The model under review builds one solid part; all positions refer to its coordinate system, in mm. A direction names the side the tool comes from. Coordinates: 2 decimals unless noted, no trailing zeros. Write each loop counter-clockwise with the first axis right and the second up, starting at its lowest first coordinate (ties: lowest second). Pieces come first, ordered by that corner, then holes. Notation, with made-up numbers: (84, 82.5) - (100, 82.5) arc R23 ccw to (100, 117.5) - close; hole circle Ø4 at (75, 23.25). An arc over 180 degrees is marked (long way). Put each result on its own line as item: value.
from build123d import *

# Parameters (mm, degrees)
SKETCH2_R           = 2.95
SKETCH2_R_2         = 8.099999999
BOSS_EXTRUDE1_DEPTH = 1


with BuildPart() as part:
    # Sketch1 → Revolve1 (revolve)
    with BuildSketch(Plane(origin=(0, 0, 0), x_dir=(0, 0, -1), z_dir=(1, 0, 0))):
        Polygon((18, 2.05), (18, 2.4), (17.5, 2.9), (8, 2.9), (8, 4), (0, 4), (0, 2.05), align=None)
    revolve(axis=Axis((0, 0, 0), (0, 0, -1)))

    # Sketch2 → Boss-Extrude1 (add)
    with BuildSketch(Plane(origin=(0, 0, -8), x_dir=(-1, 0, 0), z_dir=(0, 0, -1))):
        with BuildLine():
            Line((9.857790067, 21.711729889), (12.493283293, 10.967026744))
            Line((12.493283293, 10.967026744), (4.275989158, -2.59150858))
            ThreePointArc((4.275989158, -2.59150858), (-2.59150858, -4.275989158), (-4.275989158, 2.59150858))
            Line((-4.275989158, 2.59150858), (-0.302187827, 9.148280777))
            ThreePointArc((-0.302187827, 9.148280777), (-7.892239666, 25.676183207), (9.857790067, 21.711729889))
        make_face()
        Circle(SKETCH2_R, mode=Mode.SUBTRACT)
        with Locations((0, 19.293781382)):
            Circle(SKETCH2_R_2, mode=Mode.SUBTRACT)
    extrude(amount=BOSS_EXTRUDE1_DEPTH)


solid = part.part
1. Consider section B-B on y = 0. State the section outline as (x, z) points.
Determined:
outline: (-5.85, -9) - (-2.95, -9) - (-2.95, -8) - (-2.9, -8) - (-2.9, -17.5) - (-2.4, -18) - (-2.05, -18) - (-2.05, 0) - (-4, 0) - (-4, -8) - (-5.85, -8) - close; (2.05, -18) - (2.4, -18) - (2.9, -17.5) - (2.9, -8) - (2.95, -8) - (2.95, -9) - (5, -9) - (5, -8) - (4, -8) - (4, 0) - (2.05, 0) - close
2. Consider section A-A on x = 7.5. State the section outline as (y, z) points.
Determined:
outline: (12.45, -9) - (16.23, -9) - (16.23, -8) - (12.45, -8) - close; (22.35, -9) - (26.13, -9) - (26.13, -8) - (22.35, -8) - close
3. Machinability: for faces 1 (the cylindrical face through (0.1, -2.9, -12.7)), 2 (the flat face through (-11.16, 16.41, -8.49)), 3 (the cylindrical face through (-3.905, -0.867, -3.944)), which of the approach directions +Z, -Z, +X, -X, +Y, -Y give a long, thin tool a straight path to every point of the face, cutting with its end or side? Answer none if there is none.
Determined:
face 1: -Z
face 2: +Z, -Z, -X, +Y
face 3: +Z
4. To check wall thickness, follow probe 1 along X at (y, z) = (0, -3.75); probe 2 along X at (y, z) = (0, -14); probe 3 along Z at (x, y) = (-4.5, 4.5). State the ranges of each line that lie inside material, in increasing order.
Determined:
probe 1: x = -4 to -2.05, 2.05 to 4
probe 2: x = -2.9 to -2.05, 2.05 to 2.9
probe 3: z = -9 to -8
5. For pin 1 Ø1.5 at (x, y) = (5.5, 25) entering from +Z; pin 2 Ø2 at (x, z) = (4, -6) entering from +Y; pin 3 Ø6 at (x, z) = (1.5, -14.5) entering from -Y; pin 4 Ø2.5 at (x, y) = (0, 0) entering from -Z, all flat-tipped, find the tip position at first contact; note any pin that passes through.
Determined:
pin 1: stops at z = -8
pin 2: stops at y = 2.65
pin 3: stops at y = -2.9
pin 4: passes through
6. Consider section D-D on y = 20.5. State the section outline as (x, z) points (3 decimals), plus the area to 3 significant figures.
Determined:
outline: (-10.155, -9) - (-8.01, -9) - (-8.01, -8) - (-10.155, -8) - close; (8.01, -9) - (10.078, -9) - (10.078, -8) - (8.01, -8) - close
area: 4.21 mm^2
7. The part is to be moulded in two halves that separate along X. For faces 4 (the flat face through (1, -2, -18)), 5 (the cylindrical face through (1.054, 27.325, -8.493)), 6 (the cylindrical face through (2.033, -0.267, -9.126)), 7 (the flat face through (2.32, 5.82, -8.49)), say which applies: +X half, -X half, draft (parallel to the pull), parting line (faces both ways), or undercut.
Determined:
face 4: draft
face 5: undercut
face 6: undercut
face 7: +X half
8. Consider section C-C on z = -3. State the section outline as (x, y) points, plus the area to 3 significant figures.
Determined:
outline: circle Ø8 at (0, 0); hole circle Ø4.1 at (0, 0)
area: 37.1 mm^2
